Verification items for the finished model (mm, model axes). Face numbers are marked on the shaded views. A direction names the side the tool comes from. Give positions to 0.01 mm unless a question says otherwise; leave off trailing zeros. Order: outer loops, then holes, each group sorted by start corner. A loop starts at its lowest first (then second) coordinate and runs counter-clockwise, first axis right, second up. Notation, with made-up numbers: (33.25, 73) -> (52.25, 73) arc R25 ccw to (52.25, 100) -> close; hole circle Ø7 at (24.25, 36). An arc over 180 degrees is marked (long way). One line per question, with ' | ' between items. Start each with the question number.
Q1. Go/stop test with flat-tipped pins: pin 1 (6 mm diameter, centred on x = 9, z = 30, fed in from +Y); pin 2 (2 mm diameter, centred on x = -8, z = 26.5, fed in from +Y) (3 decimals); pin 3 (3 mm diameter, centred on y = 7.5, z = 28.5, fed in from +X). Record where each tip stops, or that it passes through.
Q2. Section check A-A on x = 0. Record the cut outline in (y, z).
Q3. Section check D-D on z = 31. Record the cut outline in (x, y), plus the area to 3 significant figures.
Q4. Section check C-C on z = 42. Record the cut outline in (x, y).
Q5. Access from +Z, -Z, +X, -X, +Y, -Y to the whole of each face (thin tool, end or side, straight path). Record for the marked faces 1, 2 and 3.
Q6. Material ranges on probe 1 along Y at (x, z) = (-0.5, 33); probe 2 along Z at (x, y) = (-14, 13); probe 3 along Y at (x, z) = (-2, 41), recorded low to high. Write a range as [from, to].
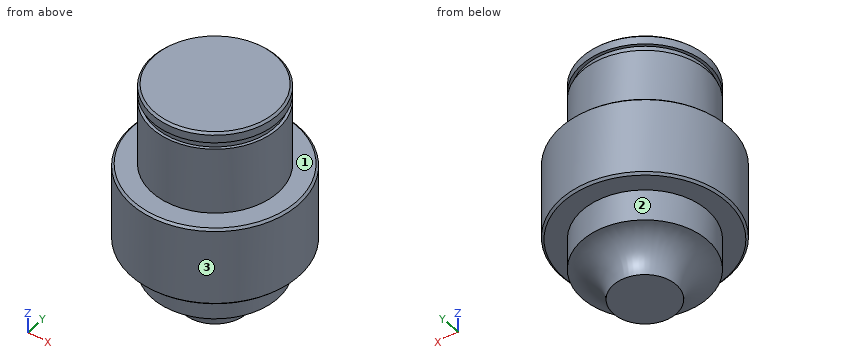
from build123d import *

# Parameters (mm, degrees)
F2_SIZE = 0.5


with BuildPart() as f1:
    # F0 (on Front) → F1 (revolve)
    with BuildSketch(Plane.XZ):
        with BuildLine():
            Line((15, 54), (0, 54))
            Line((0, 54), (0, 0))
            Line((0, 0), (7.5, 0))
            ThreePointArc((7.5, 0), (9.696699, 5.303301), (15, 7.5))
            Line((15, 7.5), (15, 15))
            Line((15, 15), (20, 15))
            Line((20, 15), (20, 34))
            Line((20, 34), (15, 34))
            Line((15, 34), (15, 50))
            Line((15, 50), (14.3, 50))
            Line((14.3, 50), (14.3, 51.6))
            Line((14.3, 51.6), (15, 51.6))
            Line((15, 51.6), (15, 54))
        make_face()
    revolve(axis=Axis((0, 0, 27), (0, 0, 1)))

    # F2
    f2_edges = [f1.edges().sort_by_distance(p)[0] for p in [
        (-15, 0, 54),
        (-20, 0, 34),
        (-20, 0, 15),
    ]]
    chamfer(f2_edges, length=F2_SIZE)


solid = f1.part
Filled in:
1) pin 1: y = 19.08 | pin 2: y = 18.735 | pin 3: x = 19.08
2) outline: (-20, 15.5) -> (-19.5, 15) -> (-15, 15) -> (-15, 7.5) arc R7.5 cw to (-7.5, 0) -> (7.5, 0) arc R7.5 cw to (15, 7.5) -> (15, 15) -> (19.5, 15) -> (20, 15.5) -> (20, 33.5) -> (19.5, 34) -> (15, 34) -> (15, 50) -> (14.3, 50) -> (14.3, 51.6) -> (15, 51.6) -> (15, 53.5) -> (14.5, 54) -> (-14.5, 54) -> (-15, 53.5) -> (-15, 51.6) -> (-14.3, 51.6) -> (-14.3, 50) -> (-15, 50) -> (-15, 34) -> (-19.5, 34) -> (-20, 33.5) -> close
3) outline: circle Ø40 at (0, 0) | area: 1,260 mm²
4) outline: circle Ø30 at (0, 0)
5) face 1: +Z | face 2: -Z | face 3: +Z, -Z
6) probe 1: [-19.99, 19.99] | probe 2: [15, 34] | probe 3: [-14.87, 14.87]
